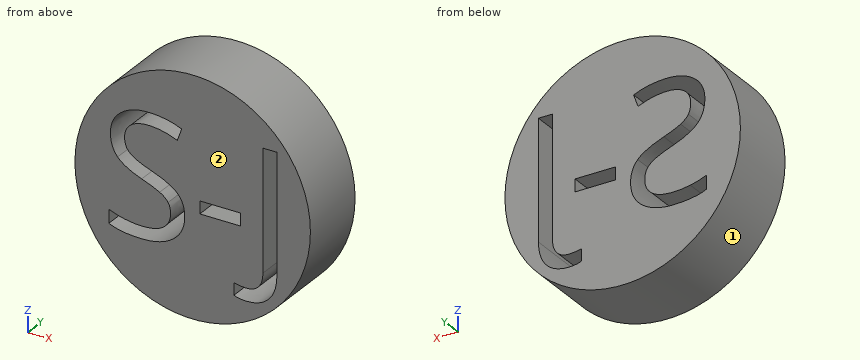
```python
from build123d import *

# Parameters (mm, degrees)
F0_R     = 41.8452571416
F0_W     = 14.3901980304
F0_H     = 4.4558957395
F1_DEPTH = 25.4


with BuildPart() as f1:
    # F0 (on Front) → F1 (new body)
    with BuildSketch(Plane.XZ):
        Circle(F0_R)
        with Locations((9.7271105858, -2.8357197633)):
            Rectangle(F0_W, F0_H, mode=Mode.SUBTRACT)
        with BuildLine():
            add(Edge.make_bspline(
                [(27.1191752197, -27.1508392515), (24.304925279, -30.2136812703), (19.0235162235, -30.2136812703)],
                knots=[0, 0, 0, 1, 1, 1], degree=2))
            add(Edge.make_bspline(
                [(19.0235162235, -30.2136812703), (16.2749321147, -30.2136812703), (14.6895713147, -29.4256912869)],
                knots=[0, 0, 0, 1, 1, 1], degree=2))
            Line((14.6895713147, -29.4256912869), (14.6895713147, -25.1761738764))
            add(Edge.make_bspline(
                [(14.6895713147, -25.1761738764), (16.7721162709, -25.7577855308), (19.0235162235, -25.7577855308)],
                knots=[0, 0, 0, 1, 1, 1], degree=2))
            add(Edge.make_bspline(
                [(19.0235162235, -25.7577855308), (21.9315744956, -25.7577855308), (23.4418886305, -23.9988793178)],
                knots=[0, 0, 0, 1, 1, 1], degree=2))
            add(Edge.make_bspline(
                [(23.4418886305, -23.9988793178), (24.9522027653, -22.2399731049), (24.9522027653, -18.9285390079)],
                knots=[0, 0, 0, 1, 1, 1], degree=2))
            Line((24.9522027653, -18.9285390079), (24.9522027653, 23.9324875899))
            Line((24.9522027653, 23.9324875899), (29.9334251605, 23.9324875899))
            Line((29.9334251605, 23.9324875899), (29.9334251605, -18.5157823499))
            add(Edge.make_bspline(
                [(29.9334251605, -18.5157823499), (29.9334251605, -24.0879972326), (27.1191752197, -27.1508392515)],
                knots=[0, 0, 0, 1, 1, 1], degree=2))
        make_face(mode=Mode.SUBTRACT)
        with BuildLine():
            add(Edge.make_bspline(
                [(-5.3478882635, -0.3732510652), (-2.8150633168, -3.1312160071), (-2.8150633168, -7.5214459147)],
                knots=[0, 0, 0, 1, 1, 1], degree=2))
            add(Edge.make_bspline(
                [(-2.8150633168, -7.5214459147), (-2.8150633168, -13.1780882956), (-6.9191778138, -16.3488098955)],
                knots=[0, 0, 0, 1, 1, 1], degree=2))
            add(Edge.make_bspline(
                [(-6.9191778138, -16.3488098955), (-11.0232923107, -19.5195314955), (-18.0589171626, -19.5195314955)],
                knots=[0, 0, 0, 1, 1, 1], degree=2))
            add(Edge.make_bspline(
                [(-18.0589171626, -19.5195314955), (-25.6761536689, -19.5195314955), (-29.7849585824, -17.5495565369)],
                knots=[0, 0, 0, 1, 1, 1], degree=2))
            Line((-29.7849585824, -17.5495565369), (-29.7849585824, -12.7465699714))
            add(Edge.make_bspline(
                [(-29.7849585824, -12.7465699714), (-27.1395636381, -13.8535082814), (-24.0345078702, -14.5007857678)],
                knots=[0, 0, 0, 1, 1, 1], degree=2))
            add(Edge.make_bspline(
                [(-24.0345078702, -14.5007857678), (-20.9294521022, -15.1480632541), (-17.880681333, -15.1480632541)],
                knots=[0, 0, 0, 1, 1, 1], degree=2))
            add(Edge.make_bspline(
                [(-17.880681333, -15.1480632541), (-12.8994589379, -15.1480632541), (-10.3760148243, -13.2578253773)],
                knots=[0, 0, 0, 1, 1, 1], degree=2))
            add(Edge.make_bspline(
                [(-10.3760148243, -13.2578253773), (-7.8525707108, -11.3675875004), (-7.8525707108, -7.9904875715)],
                knots=[0, 0, 0, 1, 1, 1], degree=2))
            add(Edge.make_bspline(
                [(-7.8525707108, -7.9904875715), (-7.8525707108, -5.7672301183), (-8.7484402753, -4.3460338982)],
                knots=[0, 0, 0, 1, 1, 1], degree=2))
            add(Edge.make_bspline(
                [(-8.7484402753, -4.3460338982), (-9.6443098397, -2.9248376781), (-11.7409260456, -1.7194006202)],
                knots=[0, 0, 0, 1, 1, 1], degree=2))
            add(Edge.make_bspline(
                [(-11.7409260456, -1.7194006202), (-13.8375422515, -0.5139635622), (-18.1152021614, 1.0057314058)],
                knots=[0, 0, 0, 1, 1, 1], degree=2))
            add(Edge.make_bspline(
                [(-18.1152021614, 1.0057314058), (-24.090792869, 3.1445613608), (-26.6564507316, 6.0760717157)],
                knots=[0, 0, 0, 1, 1, 1], degree=2))
            add(Edge.make_bspline(
                [(-26.6564507316, 6.0760717157), (-29.2221085943, 9.0075820707), (-29.2221085943, 13.726141138)],
                knots=[0, 0, 0, 1, 1, 1], degree=2))
            add(Edge.make_bspline(
                [(-29.2221085943, 13.726141138), (-29.2221085943, 18.6792210338), (-25.5026082559, 21.6107313887)],
                knots=[0, 0, 0, 1, 1, 1], degree=2))
            add(Edge.make_bspline(
                [(-25.5026082559, 21.6107313887), (-21.7831079175, 24.5422417437), (-15.6480430467, 24.5422417437)],
                knots=[0, 0, 0, 1, 1, 1], degree=2))
            add(Edge.make_bspline(
                [(-15.6480430467, 24.5422417437), (-9.2596956812, 24.5422417437), (-3.8938591275, 22.1970334597)],
                knots=[0, 0, 0, 1, 1, 1], degree=2))
            Line((-3.8938591275, 22.1970334597), (-5.451077428, 17.863088551))
            add(Edge.make_bspline(
                [(-5.451077428, 17.863088551), (-10.7606289829, 20.0863460042), (-15.7699938775, 20.0863460042)],
                knots=[0, 0, 0, 1, 1, 1], degree=2))
            add(Edge.make_bspline(
                [(-15.7699938775, 20.0863460042), (-19.7287054608, 20.0863460042), (-21.9566533306, 18.3884152066)],
                knots=[0, 0, 0, 1, 1, 1], degree=2))
            add(Edge.make_bspline(
                [(-21.9566533306, 18.3884152066), (-24.1846012003, 16.690484409), (-24.1846012003, 13.6698561392)],
                knots=[0, 0, 0, 1, 1, 1], degree=2))
            add(Edge.make_bspline(
                [(-24.1846012003, 13.6698561392), (-24.1846012003, 11.446598686), (-23.3637783009, 10.0207120494)],
                knots=[0, 0, 0, 1, 1, 1], degree=2))
            add(Edge.make_bspline(
                [(-23.3637783009, 10.0207120494), (-22.5429554016, 8.5948254127), (-20.5917421093, 7.408150021)],
                knots=[0, 0, 0, 1, 1, 1], degree=2))
            add(Edge.make_bspline(
                [(-20.5917421093, 7.408150021), (-18.640528817, 6.2214746294), (-14.6255322349, 4.7862071596)],
                knots=[0, 0, 0, 1, 1, 1], degree=2))
            add(Edge.make_bspline(
                [(-14.6255322349, 4.7862071596), (-7.8807132102, 2.3847138768), (-5.3478882635, -0.3732510652)],
                knots=[0, 0, 0, 1, 1, 1], degree=2))
        make_face(mode=Mode.SUBTRACT)
    extrude(amount=F1_DEPTH)


solid = f1.part
```
Input: part model. Units: mm. Frame: model coordinates. Face numbers are marked on the shaded views. Give positions to 0.01 mm unless a question says otherwise; leave off trailing zeros. Loops run counter-clockwise (first coordinate to the right, second up) from the corner with the lowest first, then second, coordinate; pieces in that order, holes last.
1) Section query B-B on y = -14.5. Count the separate pieces of the cut face and the enclosed holes in it, and give its area (3 significant figures).
A:
separate pieces: 1
enclosed holes: 3
area: 4,710 mm2
2) Line query: L1, parallel to X at y = -17.75, z = -1.5; L2, parallel to X at y = -4, z = 12.5; L3, parallel to X at y = -8.5, z = 2. Output: solid intervals per line, ascending.
A:
L1: x = -41.82 to -12.14, -4.46 to 2.53, 16.92 to 24.95, 29.93 to 41.82
L2: x = -39.93 to -29.18, -24.12 to 24.95, 29.93 to 39.93
L3: x = -41.8 to -20.61, -8.42 to 24.95, 29.93 to 41.8
3) Mould query, pull axis X, two halves, no side actions, for the marked faces 1 and 2. Classes: released by +X, released by -X, zero draft, split by the parting line, or undercut.
A:
face 1: split by the parting line
face 2: zero draft
4) Contact query for flat-ended pins moving along their axis: pin 1 (4 mm diameter, centred on x = 28, y = -13, fed in from -Z); pin 2 (1 mm diameter, centred on y = -21, z = 28.5, fed in from -X); pin 3 (2 mm diameter, centred on y = -4.5, z = 13, fed in from +X); pin 4 (8 mm diameter, centred on x = 5, z = -29, fed in from +Y). Output: stop coordinate, or through.
A:
pin 1: stops at z = -32.79
pin 2: stops at x = -31.1
pin 3: stops at x = 40.09
pin 4: stops at y = 0
5) Section query A-A on x = 4. Return the cut outline in (y, z).
A:
outline: (-25.4, -41.65) - (0, -41.65) - (0, -5.06) - (-25.4, -5.06) - close; (-25.4, -0.61) - (0, -0.61) - (0, 41.65) - (-25.4, 41.65) - close
